Verification items for the finished model (mm, model axes). A direction names the side the tool comes from. Coordinates: 2 decimals unless noted, no trailing zeros. Write each loop counter-clockwise with the first axis right and the second up, starting at its lowest first coordinate (ties: lowest second). Pieces come first, ordered by that corner, then holes. Notation, with made-up numbers: (67, 62.25) - (80, 62.25) arc R20 ccw to (80, 87.25) - close; hole circle Ø6 at (26, -26). An arc over 180 degrees is marked (long way). Answer as CSV lines item,"result". Start each with the question number.
```python
from build123d import *

# Parameters (mm, degrees)
F0_W     = 1930.4
F0_H     = 2032
F1_DEPTH = 254
F2_W     = 1828.8
F2_H     = 1930.4
F2_W_2   = 1778
F2_H_2   = 1879.6
F3_DEPTH = 152.4
F4_R     = 25.4


with BuildPart() as f1:
    # F0 (on Top) → F1 (new body)
    with BuildSketch(Plane.XY):
        with Locations((-34.384124, -14.047471)):
            Rectangle(F0_W, F0_H)
    extrude(amount=-F1_DEPTH)

    # F2 (on face) → F3 (join)
    with BuildSketch(Plane(origin=(0, 0, -254), x_dir=(1, 0, 0), z_dir=(0, 0, -1))):
        with Locations((-34.384124, 14.047471)):
            Rectangle(F2_W, F2_H)
        with Locations((-34.384124, 14.047471)):
            Rectangle(F2_W_2, F2_H_2, mode=Mode.SUBTRACT)
    extrude(amount=F3_DEPTH)

    # F4
    f4_edges = [f1.edges().sort_by_distance(p)[0] for p in [
        (-999.584124, 1001.952529, -127),
        (-999.584124, -1030.047471, -127),
        (-999.584124, -14.047471, 0),
        (-999.584124, -14.047471, -254),
        (930.815876, 1001.952529, -127),
        (-34.384124, 1001.952529, 0),
        (-34.384124, 1001.952529, -254),
        (930.815876, -1030.047471, -127),
        (930.815876, -14.047471, 0),
        (930.815876, -14.047471, -254),
        (-34.384124, -1030.047471, 0),
        (-34.384124, -1030.047471, -254),
        (880.015876, -979.247471, -330.2),
        (880.015876, 951.152529, -330.2),
        (-948.784124, 951.152529, -330.2),
        (-948.784124, -979.247471, -330.2),
    ]]
    fillet(f4_edges, radius=F4_R)


solid = f1.part
```
1. Cross-section at B-B (x = -670). Record the cut outline in (y, z), and give its area (3 significant figures).
2. Cross-section at A-A (z = -324). Record the cut outline in (x, y).
3. Cross-section at C-C (y = 450.5). Record the cut outline in (x, z), and give its area (3 significant figures).
4. Scan lines: line 1 along X through (y, z) = (332, -357); line 2 along Y through (x, z) = (594.5, -388); line 3 along Z through (x, y) = (184, -665.5). Record each from-to range of solid material in increasing order. Write a range as from..to.
5. Access from +Z, -Z, +X, -X, +Y, -Y to the whole of each face (thin tool, end or side, straight path). Record for faces 5 (the face through (-47, -979.247, -329)), 6 (the face through (854.616, -1, -329)), 7 (the face through (-47, 951.153, -329)), 8 (the face through (880.016, -1, -329)).
6. Draft check along X on faces 1 (the face through (-48, 0, 0)), 2 (the face through (-948.784, -1, -329)), 3 (the face through (-47, 925.753, -329)), 4 (the face through (-47, -1, -254)). Enter one of: pulls with the +X half, pulls with the -X half, needs draft (parallel to the pull), parting line crosses it, or undercut.
7. Depth check by flat-ended pin: P1, Ø6, axis at y = -36, z = -351, coming from the -X side; P2, Ø3, axis at x = 191.5, z = -280, coming from the +Y side. Enter the tip coordinate at first touch or a pass-through.
Completed:
1,outline,"(-1030.05, -228.6) arc R25.4 ccw to (-1004.65, -254) - (-979.25, -254) - (-979.25, -406.4) - (-953.85, -406.4) - (-953.85, -254) - (925.75, -254) - (925.75, -406.4) - (951.15, -406.4) - (951.15, -254) - (976.55, -254) arc R25.4 ccw to (1001.95, -228.6) - (1001.95, -25.4) arc R25.4 ccw to (976.55, 0) - (-1004.65, 0) arc R25.4 ccw to (-1030.05, -25.4) - close"
1,area,"523,000 mm2"
2,outline,"(-948.78, -953.85) arc R25.4 ccw to (-923.38, -979.25) - (854.62, -979.25) arc R25.4 ccw to (880.02, -953.85) - (880.02, 925.75) arc R25.4 ccw to (854.62, 951.15) - (-923.38, 951.15) arc R25.4 ccw to (-948.78, 925.75) - close; hole (-923.38, -953.85) - (854.62, -953.85) - (854.62, 925.75) - (-923.38, 925.75) - close"
3,outline,"(-999.58, -228.6) arc R25.4 ccw to (-974.18, -254) - (-948.78, -254) - (-948.78, -406.4) - (-923.38, -406.4) - (-923.38, -254) - (854.62, -254) - (854.62, -406.4) - (880.02, -406.4) - (880.02, -254) - (905.42, -254) arc R25.4 ccw to (930.82, -228.6) - (930.82, -25.4) arc R25.4 ccw to (905.42, 0) - (-974.18, 0) arc R25.4 ccw to (-999.58, -25.4) - close"
3,area,"498,000 mm2"
4,line 1,"x = -948.78..-923.38, 854.62..880.02"
4,line 2,"y = -979.25..-953.85, 925.75..951.15"
4,line 3,"z = -254..0"
5,face 5,"-Z, +X, -X, -Y"
5,face 6,"-Z"
5,face 7,"-Z, +X, -X, +Y"
5,face 8,"-Z, +X, +Y, -Y"
6,face 1,"needs draft"
6,face 2,"pulls with the -X half"
6,face 3,"undercut"
6,face 4,"undercut"
7,P1,"stops at x = -948.78"
7,P2,"stops at y = 951.15"
